CAD build for the part. Positions are in the model's coordinates, mm. A direction names the side the tool comes from. Coordinates: 2 decimals unless noted, no trailing zeros. Order: outer loops, then holes, each group sorted by start corner. A loop starts at its lowest first (then second) coordinate and runs counter-clockwise, first axis right, second up. Notation, with made-up numbers: (2, -5) -> (39, -5) arc R19 ccw to (39, 31) -> close; hole circle Ø4 at (-20, 59). An arc over 180 degrees is marked (long way). Use one line per item in the form item = value. Start each with the question number.
from build123d import *

# Parameters (mm, degrees)
F1_DEPTH = 63.5
F2_SIZE  = 0.508


with BuildPart() as f1:
    # F0 (on Front) → F1 (new body)
    with BuildSketch(Plane.XZ):
        with BuildLine():
            ThreePointArc((0, 4.7625), (1.3949039546, 1.3949039546), (4.7625, 0))
            Line((4.7625, 0), (17.4625, 0))
            Line((17.4625, 0), (17.4625, 3.175))
            Line((17.4625, 3.175), (20.6375, 3.175))
            Line((20.6375, 3.175), (20.6375, 0))
            Line((20.6375, 0), (34.925, 0))
            Line((34.925, 0), (34.925, 6.35))
            Line((34.925, 6.35), (10.795, 6.35))
            Line((10.795, 6.35), (10.795, 12.7))
            Line((10.795, 12.7), (4.7625, 12.7))
            ThreePointArc((4.7625, 12.7), (1.3949039546, 11.3050960454), (0, 7.9375))
            Line((0, 7.9375), (0, 4.7625))
        make_face()
    extrude(amount=F1_DEPTH)

    # F2
    f2_edges = [f1.edges().sort_by_distance(p)[0] for p in [
        (10.795, -31.75, 12.7),
    ]]
    chamfer(f2_edges, length=F2_SIZE)


solid = f1.part
1) Two-plate mould, pull along X, no slides. Class faces 1 (the face through (28, -31, 0)), 2 (the face through (19, -31, 3.175)), 3 (the face through (20.638, -31, 2)), 4 (the face through (10.795, -31, 9)): released by +X, released by -X, zero draft, split by the parting line, or undercut.
2) 3-axis set-ups, long thin cutter, end or side, ignore diameter. For faces 5 (the face through (13, 0, 5)), 6 (the face through (23, -31, 6.35)), 7 (the face through (17.462, -31, 2)): which of +Z, -Z, +X, -X, +Y, -Y reach the whole face in a straight line?
3) Cut at C-C on x = 23.5. Give the cut face in (y, z).
4) Drop flat-ended pins along their axis: P1, Ø1, axis at y = -40, z = 4, coming from the -X side; P2, Ø3.5, axis at y = -47.5, z = 1, coming from the -X side; P3, Ø1, axis at x = 21, y = -35.5, coming from the +Z side. Give the stop position or say it passes through.
5) Cut at B-B on z = 2.25. Give the cut face in (x, y) (1 decimal), then the cut area to 3 significant figures.
6) Cut at D-D on z = 7. Give the cut face in (x, y) (3 decimals).
7) Probe L1, parallel to Z at x = 21, y = -36; L2, parallel to X at y = -38, z = 2.5 (1 decimal); L3, parallel to X at y = -44, z = 6.75 (3 decimals). List the from-to ranges inside material, lowest first.
Values follow:
q1.face_1 = zero draft
q1.face_2 = undercut
q1.face_3 = undercut
q1.face_4 = released by +X
q2.face_5 = +Z, -Z, +X, -X, +Y
q2.face_6 = +Z, +X, +Y, -Y
q2.face_7 = -Z, +Y, -Y
q3.outline = (-63.5, 0) -> (0, 0) -> (0, 6.35) -> (-63.5, 6.35) -> close
q4.P1 = 0.01
q4.P2 = 0.45
q4.P3 = 6.35
q5.outline = (0.7, -63.5) -> (17.5, -63.5) -> (17.5, 0) -> (0.7, 0) -> close; (20.6, -63.5) -> (34.9, -63.5) -> (34.9, 0) -> (20.6, 0) -> close
q5.area = 1,970 mm^2
q6.outline = (0, -63.5) -> (10.795, -63.5) -> (10.795, 0) -> (0, 0) -> close
q7.L1 = 0 to 6.35
q7.L2 = 0.6 to 17.5, 20.6 to 34.9
q7.L3 = 0 to 10.795
